Source: CAD feature listing. Evaluate the final solid. Frame: model axes, mm. Face numbers are marked on the shaded views. A direction names the side the tool comes from. Give positions to 0.01 mm unless a question says otherwise; leave off trailing zeros. Order: outer loops, then holes, each group sorted by start corner. A loop starts at its lowest first (then second) coordinate and runs counter-clockwise, first axis right, second up. Notation, with made-up numbers: (48, -16.75) - (96, -16.75) arc R15 ccw to (96, -11.75) - close; hole circle Ø8 at (89.5, 31.5). An arc over 180 degrees is marked (long way). Use CSV: the item, a comma, the result in double quotes.
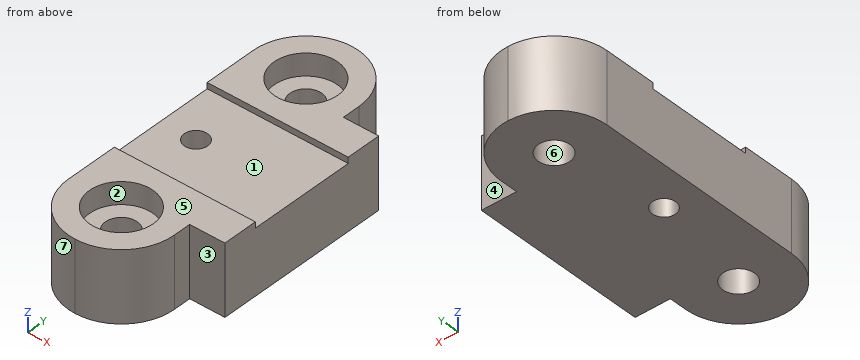
```python
from build123d import *

# Parameters (mm, degrees)
AUFSATZ_LINEAR_AUSTRAGEN1_DEPTH                      = 10
SKIZZE2_W                                            = 20
SKIZZE2_H                                            = 15.1
SCHNITT_LINEAR_AUSTRAGEN1_DEPTH                      = 0.85
STIRNSENKUNG_F_R_M4_FLACHKOPFSCHRAUBE_MI_D           = 4.5
STIRNSENKUNG_F_R_M4_FLACHKOPFSCHRAUBE_MI_CBORE_D     = 9
STIRNSENKUNG_F_R_M4_FLACHKOPFSCHRAUBE_MI_CBORE_DEPTH = 3.1
M4_GEWINDEBOHRUNG1_D                                 = 3.3
VERRUNDUNG1_R                                        = 7.5


with BuildPart() as part:
    # Skizze1 → Aufsatz-Linear austragen1 (new body)
    with BuildSketch(Plane.XY):
        Polygon((0, 0), (0, 45), (15, 45), (15, 35), (20, 35), (20, 10), (15, 10), (15, 0), align=None)
    extrude(amount=AUFSATZ_LINEAR_AUSTRAGEN1_DEPTH)

    # Skizze2 → Schnitt-Linear austragen1 (cut)
    with BuildSketch(Plane.XY.offset(10)):
        with Locations((10, 22.5)):
            Rectangle(SKIZZE2_W, SKIZZE2_H)
    extrude(amount=-SCHNITT_LINEAR_AUSTRAGEN1_DEPTH, mode=Mode.SUBTRACT)

    # Stirnsenkung für M4 Flachkopfschraube mit Schlitz1 (through all)
    with Locations(Plane.XY.offset(10)):
        with Locations((7.5, 37.5), (7.5, 7.5)):
            CounterBoreHole(STIRNSENKUNG_F_R_M4_FLACHKOPFSCHRAUBE_MI_D / 2, STIRNSENKUNG_F_R_M4_FLACHKOPFSCHRAUBE_MI_CBORE_D / 2, STIRNSENKUNG_F_R_M4_FLACHKOPFSCHRAUBE_MI_CBORE_DEPTH)

    # M4 Gewindebohrung1 (through all)
    with Locations(Plane.XY.offset(9.15)):
        with Locations((5, 22.5)):
            Hole(M4_GEWINDEBOHRUNG1_D / 2)

    # Verrundung1
    verrundung1_edges = [part.edges().sort_by_distance(p)[0] for p in [
        (0, 0, 5),
        (15, 0, 5),
        (15, 45, 5),
        (0, 45, 5),
    ]]
    fillet(verrundung1_edges, radius=VERRUNDUNG1_R - 0.0001)  # a hair under: the kernel refuses the full size


solid = part.part
```
Item 1: Section C-C on x = 18.5. Return the cut outline in (y, z).
Filled in:
outline,"(10, 0) - (35, 0) - (35, 10) - (30.05, 10) - (30.05, 9.15) - (14.95, 9.15) - (14.95, 10) - (10, 10) - close"
Item 2: Section B-B on y = 22.5. Return the cut outline in (x, z), then the cut area to 3 significant figures.
Filled in:
outline,"(0, 0) - (3.35, 0) - (3.35, 9.15) - (0, 9.15) - close; (6.65, 0) - (20, 0) - (20, 9.15) - (6.65, 9.15) - close"
area,"153 mm2"
Item 3: Section A-A on z = 6. Count the separate pieces of the cut face and the enclosed holes in it, then the cut area to 3 significant figures.
Filled in:
separate pieces,"1"
enclosed holes,"3"
area,"711 mm2"
Item 4: Material intervals for line 1 (Y direction, x = 7.5, z = 9.75); line 2 (Y direction, x = 7.5, z = 2.25); line 3 (Y direction, x = 7.5, z = 9.05), sorted ascending. Write a range as from..to.
Filled in:
line 1,"y = 0..3, 12..14.95, 30.05..33, 42..45"
line 2,"y = 0..5.25, 9.75..35.25, 39.75..45"
line 3,"y = 0..3, 12..33, 42..45"
Item 5: Set-up query: the marked faces 1, 2, 3 and 4. Return all of +Z, -Z, +X, -X, +Y, -Y with unobstructed straight access to the full face (end or side cutting, diameter ignored); none if empty.
Filled in:
face 1,"+Z, +X, -X"
face 2,"+Z"
face 3,"+Z, -Z, +X, -Y"
face 4,"+Z, -Z, +X, +Y"
Item 6: First-contact query: pin 1 (4 mm diameter, centred on x = 14, z = 8, fed in from +Y); pin 2 (8 mm diameter, centred on x = 4, y = 8, fed in from -Z); pin 3 (2.5 mm diameter, centred on x = 18.5, z = 3, fed in from +Y); pin 4 (5.5 mm diameter, centred on x = 16.5, z = 3, fed in from -Y). Flat tips, straight axial feed; report the tip coordinate or a pass-through.
Filled in:
pin 1,"stops at y = 43.5"
pin 2,"stops at z = 0"
pin 3,"stops at y = 35"
pin 4,"stops at y = 3.35"
Item 7: Mould query, pull axis Y, two halves, no side actions, for the marked faces 5, 6 and 7. Classes: released by +Y, released by -Y, zero draft, split by the parting line, or undercut.
Filled in:
face 5,"zero draft"
face 6,"undercut"
face 7,"released by -Y"
Item 8: Section D-D on y = 4. Return the cut outline in (x, z), then the cut area to 3 significant figures.
Filled in:
outline,"(0.87, 0) - (14.13, 0) - (14.13, 10) - (10.33, 10) - (10.33, 6.9) - (4.67, 6.9) - (4.67, 10) - (0.87, 10) - close"
area,"115 mm2"
